from build123d import *

# Parameters (mm, degrees)
CHAMFER2_SIZE     = 0.3
CIRPATTERN1_COUNT = 2
FILLET2_R         = 0.2
FILLET3_R         = 1


with BuildPart() as part:
    # Sketch1 → Revolve1 (revolve)
    with BuildSketch(Plane.XY, mode=Mode.PRIVATE) as revolve1_sk:
        Polygon((0, 0), (-7.25, 0), (-7.25, 3.5), (-3.1, 3.5), (-3.1, 1), (0, 1), align=None)
    revolve(revolve1_sk.sketch.rotate(Axis((0, 0, 0), (0, 1, 0)), 270), axis=Axis((0, 0, 0), (0, 1, 0)))

    # Chamfer2
    chamfer2_edges = [part.edges().sort_by_distance(p)[0] for p in [
        (0, 3.5, 3.1),
    ]]
    chamfer(chamfer2_edges, length=CHAMFER2_SIZE)

    # Sketch4 → CSK for M2 Flat Head Machine Screw1 (revolve, cut)
    with BuildSketch(Plane(origin=(-4.75, 0, 0), x_dir=(0, 0, -1), z_dir=(1, 0, 0))):
        Polygon((0, 0), (0, 5.660946681), (1.1, 5), (1.1, 1.1), (2.2, 0), align=None)
    csk_for_m2_flat_head_machine_screw1 = revolve(axis=Axis((-4.75, -6.35, 0), (0, 1, 0)), mode=Mode.SUBTRACT)

    # CirPattern1: CSK for M2 Flat Head Machine Screw1 ×2 about axis
    cirpattern1_axis = Axis((0, 0, 0), (0, 1, 0))
    for i in range(1, CIRPATTERN1_COUNT):
        add(csk_for_m2_flat_head_machine_screw1.rotate(cirpattern1_axis, i * 360 / CIRPATTERN1_COUNT), mode=Mode.SUBTRACT)

    # Fillet2
    fillet2_edges = [part.edges().sort_by_distance(p)[0] for p in [
        (0, 1, 3.1),
    ]]
    fillet(fillet2_edges, radius=FILLET2_R)

    # Fillet3
    fillet3_edges = [part.edges().sort_by_distance(p)[0] for p in [
        (0, 3.5, 7.25),
    ]]
    fillet(fillet3_edges, radius=FILLET3_R)


solid = part.part
Geometry check sheet. Reference: the model listing, model coordinates, mm. A direction names the side the tool comes from. Give positions to 0.01 mm unless a question says otherwise; leave off trailing zeros. Write each loop counter-clockwise with the first axis right and the second up, starting at its lowest first coordinate (ties: lowest second). Pieces come first, ordered by that corner, then holes.
1) Release check for a two-part mould opening along Z. For faces 3 (the face through (-5.68, 2.28, -0.59)), 4 (the face through (2.777, 1.268, -6.697)), 5 (the face through (0, 0, 0)) record: released by +Z, released by -Z, zero draft, split by the parting line, or undercut.
Values follow:
face 3: undercut
face 4: split by the parting line
face 5: zero draft
2) Go/stop test with flat-tipped pins: pin 1 Ø1.7 at (x, z) = (-0.5, 0) entering from +Y; pin 2 Ø1 at (x, y) = (-5.5, 0.5) entering from -Z; pin 3 Ø2 at (y, z) = (0.5, 1.5) entering from +X. Record where each tip stops, or that it passes through.
Values follow:
pin 1: stops at y = 1
pin 2: stops at z = -5.25
pin 3: stops at x = 7.23
3) Cross-section at C-C (y = 2.25). Record the boundary of the cut face in (x, z), plus the area to 3 significant figures.
Values follow:
outline: circle Ø14.5 at (0, 0); hole circle Ø2.2 at (-4.75, 0); hole circle Ø6.2 at (0, 0); hole circle Ø2.2 at (4.75, 0)
area: 127 mm2
4) Set-up check for faces 1 (the face through (5.68, 2.28, 0.59)), 2 (the face through (0, 1, 0)): record each of +Z, -Z, +X, -X, +Y, -Y from which the full face is reachable in a straight line by a thin tool's end or side.
Values follow:
face 1: +Y, -Y
face 2: +Y
5) Cross-section at A-A (z = 0). Record the boundary of the cut face in (x, y).
Values follow:
outline: (-7.25, 0) - (-6.95, 0) - (-5.85, 1.1) - (-5.85, 3.5) - (-6.25, 3.5) arc R1 ccw to (-7.25, 2.5) - close; (-3.65, 1.1) - (-2.55, 0) - (2.55, 0) - (3.65, 1.1) - (3.65, 3.5) - (3.4, 3.5) - (3.1, 3.2) - (3.1, 1.2) arc R0.2 cw to (2.9, 1) - (-2.9, 1) arc R0.2 cw to (-3.1, 1.2) - (-3.1, 3.2) - (-3.4, 3.5) - (-3.65, 3.5) - close; (5.85, 1.1) - (6.95, 0) - (7.25, 0) - (7.25, 2.5) arc R1 ccw to (6.25, 3.5) - (5.85, 3.5) - close
6) Cross-section at B-B (x = 0). Record the boundary of the cut face in (y, z), plus the area to 3 significant figures.
Values follow:
outline: (0, -7.25) - (2.5, -7.25) arc R1 ccw to (3.5, -6.25) - (3.5, -3.4) - (3.2, -3.1) - (1.2, -3.1) arc R0.2 cw to (1, -2.9) - (1, 2.9) arc R0.2 cw to (1.2, 3.1) - (3.2, 3.1) - (3.5, 3.4) - (3.5, 6.25) arc R1 ccw to (2.5, 7.25) - (0, 7.25) - close
area: 34.7 mm2
7) Thickness scan on line 1 (X direction, y = 2.05, z = 0); line 2 (X direction, y = 1.05, z = 1); line 3 (Y direction, x = -1.75, z = 1). Record the ranges inside material, lowest first.
Values follow:
line 1: x = -7.25 to -5.85, -3.65 to -3.1, 3.1 to 3.65, 5.85 to 7.25
line 2: x = -7.18 to -5.32, -4.18 to -2.86, 2.86 to 4.18, 5.32 to 7.18
line 3: y = 0 to 1
